Check sheet for the modelled part. Datum: model origin and axes. Units: mm. A direction names the side the tool comes from. Round coordinates to 2 decimals unless told otherwise and drop trailing zeros. Loops run counter-clockwise (first coordinate to the right, second up) from the corner with the lowest first, then second, coordinate; pieces in that order, holes last. Notation, with made-up numbers: (-9, 86) - (-2, 86) arc R4 ccw to (-2, 90) - close; hole circle Ø1 at (-6.75, 0). An arc over 180 degrees is marked (long way). Put each result on its own line as item: value. Start each with the question number.
Item 1: Draft check along Y on faces 1 (the cylindrical face through (-2.222, -10.006, 1.38)), 2 (the cylindrical face through (7.2, -0.6, 1.4)), 3 (the flat face through (2, 0, 0)). Enter one of: pulls with the +Y half, pulls with the -Y half, needs draft (parallel to the pull), parting line crosses it, or undercut.
Item 2: Section check D-D, the plane y = 8. Record the cut outline in (x, z), and give its area (3 significant figures).
Item 3: Material ranges on line 1 along Y through (x, z) = (0, 0.9); line 2 along Z through (x, y) = (-8.25, 2.25); line 3 along X through (y, z) = (-8.25, 0.3), recorded low to high.
Item 4: Section check B-B, the plane z = 1.4. Record the cut outline in (x, y).
Item 5: Section check C-C, the plane x = -0.75. Record the cut outline in (y, z), and give its area (3 significant figures).
Item 6: Section check A-A, the plane y = 0. Record the cut outline in (x, z).
Item 7: Gauge pin test, flat ends, axial feed: pin 1 Ø1.8 at (x, y) = (0, 8) entering from +Z; pin 2 Ø1 at (x, z) = (-1.5, 0.5) entering from +Y. Record the tip position at first contact, or that the pin passes through.
Item 8: Tool access check on faces 4 (the cylindrical face through (0, -7, 1)), 5 (the cylindrical face through (-0.867, -3.905, 3.293)). Record the directions out of +Z, -Z, +X, -X, +Y, -Y that give a thin tool (end or side, any length) a straight path to the whole face; none if there is none.
from build123d import *

# Parameters (mm, degrees)
SKETCH1_R           = 10.25
SKETCH1_R_2         = 4
BOSS_EXTRUDE1_DEPTH = 2.8
SKETCH1_3_R         = 4
SKETCH1_3_R_2       = 1.6
BOSS_EXTRUDE2_DEPTH = 3.8
SKETCH2_R           = 1
CUT_EXTRUDE1_DEPTH  = 2.8


with BuildPart() as part:
    # Sketch1 → Boss-Extrude1 (new body)
    with BuildSketch(Plane.XY):
        Circle(SKETCH1_R)
        Circle(SKETCH1_R_2, mode=Mode.SUBTRACT)
    extrude(amount=BOSS_EXTRUDE1_DEPTH)

    # Sketch1<3> → Boss-Extrude2 (add)
    with BuildSketch(Plane.XY):
        Circle(SKETCH1_3_R)
        Circle(SKETCH1_3_R_2, mode=Mode.SUBTRACT)
    extrude(amount=BOSS_EXTRUDE2_DEPTH)

    # Sketch2 → Cut-Extrude1 (cut)
    with BuildSketch(Plane.XY.offset(2.8)):
        with Locations((0, 8)):
            Circle(SKETCH2_R)
        with Locations((8, 0)):
            Circle(SKETCH2_R)
        with Locations((0, -8)):
            Circle(SKETCH2_R)
        with Locations((-8, 0)):
            Circle(SKETCH2_R)
    extrude(amount=-CUT_EXTRUDE1_DEPTH, mode=Mode.SUBTRACT)


solid = part.part
Check result:
1. face 1: parting line crosses it
1. face 2: undercut
1. face 3: needs draft
2. outline: (-6.41, 0) - (-1, 0) - (-1, 2.8) - (-6.41, 2.8) - close; (1, 0) - (6.41, 0) - (6.41, 2.8) - (1, 2.8) - close
2. area: 30.3 mm²
3. line 1: -10.25 to -9, -7 to -1.6, 1.6 to 7, 9 to 10.25
3. line 2: 0 to 2.8
3. line 3: -6.08 to -0.97, 0.97 to 6.08
4. outline: circle Ø20.5 at (0, 0); hole circle Ø2 at (-8, 0); hole circle Ø3.2 at (0, 0); hole circle Ø2 at (0, -8); hole circle Ø2 at (0, 8); hole circle Ø2 at (8, 0)
5. outline: (-10.22, 0) - (-8.66, 0) - (-8.66, 2.8) - (-10.22, 2.8) - close; (-7.34, 0) - (-1.41, 0) - (-1.41, 3.8) - (-3.93, 3.8) - (-3.93, 2.8) - (-7.34, 2.8) - close; (1.41, 0) - (7.34, 0) - (7.34, 2.8) - (3.93, 2.8) - (3.93, 3.8) - (1.41, 3.8) - close; (8.66, 0) - (10.22, 0) - (10.22, 2.8) - (8.66, 2.8) - close
5. area: 47.0 mm²
6. outline: (-10.25, 0) - (-9, 0) - (-9, 2.8) - (-10.25, 2.8) - close; (-7, 0) - (-1.6, 0) - (-1.6, 3.8) - (-4, 3.8) - (-4, 2.8) - (-7, 2.8) - close; (1.6, 0) - (7, 0) - (7, 2.8) - (4, 2.8) - (4, 3.8) - (1.6, 3.8) - close; (9, 0) - (10.25, 0) - (10.25, 2.8) - (9, 2.8) - close
7. pin 1: through
7. pin 2: y = 10.2
8. face 4: +Z, -Z
8. face 5: +Z
